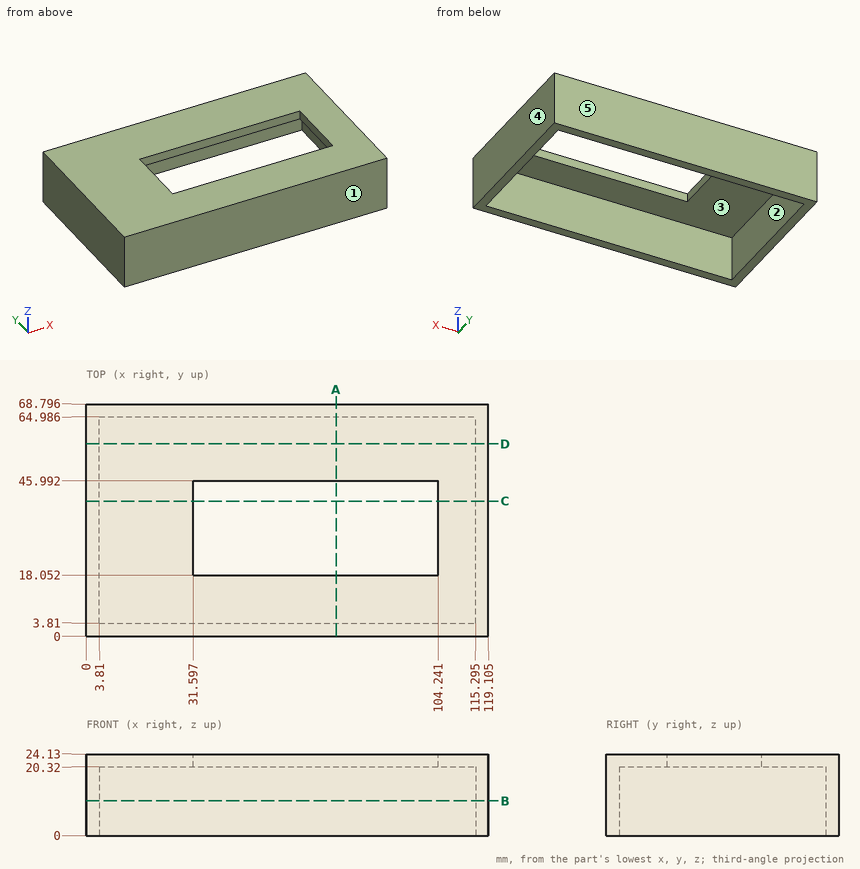
Input: dimensioned drawing with shaded views. Units: mm. Origin: part minimum x, y, z. A direction names the side the tool comes from. Coordinates: 2 decimals unless noted, no trailing zeros. Order: outer loops, then holes, each group sorted by start corner. A loop starts at its lowest first (then second) coordinate and runs counter-clockwise, first axis right, second up. Notation, with made-up numbers: (68, 49) - (100, 49) arc R16 ccw to (100, 62) - close; hole circle Ø9 at (56.25, 60). An arc over 180 degrees is marked (long way). One line per item, written item: value.
1) Contact query for a flat-ended pin moving along its axis: pin 1 (1 mm diameter, centred on x = 43.5, y = 56, fed in from -Z). Output: stop coordinate, or through.
Computed values:
pin 1: stops at z = 20.32
2) Cut plane A-A on x = 74. Output: boundary loops of the cut face in (y, z).
Computed values:
outline: (0, 0) - (3.81, 0) - (3.81, 20.32) - (18.05, 20.32) - (18.05, 24.13) - (0, 24.13) - close; (45.99, 20.32) - (64.99, 20.32) - (64.99, 0) - (68.8, 0) - (68.8, 24.13) - (45.99, 24.13) - close
3) Cut plane D-D on y = 57. Output: boundary loops of the cut face in (x, z) (1 decimal).
Computed values:
outline: (0, 0) - (3.8, 0) - (3.8, 20.3) - (115.3, 20.3) - (115.3, 0) - (119.1, 0) - (119.1, 24.1) - (0, 24.1) - close
4) Cut plane B-B on z = 10.25. Output: boundary loops of the cut face in (x, y) (1 decimal), plus the area to 3 significant figures.
Computed values:
outline: (0, 0) - (119.1, 0) - (119.1, 68.8) - (0, 68.8) - close; hole (3.8, 3.8) - (115.3, 3.8) - (115.3, 65) - (3.8, 65) - close
area: 1,370 mm^2
5) Mould query, pull axis X, two halves, no side actions, for the marked faces 3, 4 and 5. Classes: released by +X, released by -X, zero draft, split by the parting line, or undercut.
Computed values:
face 3: undercut
face 4: released by +X
face 5: zero draft
6) Reachability of the marked faces 1 and 2 from +Z, -Z, +X, -X, +Y, -Y: full face, straight path, thin tool, end or side. Return the list, or none.
Computed values:
face 1: +Z, -Z, +X, -X, -Y
face 2: -Z
7) Ray query, line 1 (X direction, y = 24.5, z = 15.75) (1 decimal); line 2 (Y direction, x = 89, z = 13.75); line 3 (X direction, y = 29.5, z = 21) (1 decimal). Return the intervals inside material, ascending. Write a range as [from, to].
Computed values:
line 1: x = [0, 3.8], [115.3, 119.1]
line 2: y = [0, 3.81], [64.99, 68.8]
line 3: x = [0, 31.6], [104.2, 119.1]
8) Cut plane C-C on y = 40. Output: boundary loops of the cut face in (x, z) (1 decimal), plus the area to 3 significant figures.
Computed values:
outline: (0, 0) - (3.8, 0) - (3.8, 20.3) - (31.6, 20.3) - (31.6, 24.1) - (0, 24.1) - close; (104.2, 20.3) - (115.3, 20.3) - (115.3, 0) - (119.1, 0) - (119.1, 24.1) - (104.2, 24.1) - close
area: 332 mm^2
